from build123d import *

# Parameters (mm, degrees)
BOSS_EXTRUDE1_DEPTH      = 33.02
BOSS_EXTRUDE1_DEPTH_BACK = 33.02
BOSS_EXTRUDE3_DEPTH      = 19.05
BOSS_EXTRUDE3_DEPTH_BACK = 19.05
SKETCH2_6_W              = 38.1
SKETCH2_6_H              = 81.28
SKETCH8_OUTSIDE_W        = 151.232
SKETCH8_OUTSIDE_H        = 112.624
SKETCH8_OUTSIDE_R        = 19.05
CUT_EXTRUDE1_DEPTH       = 81.28
CHAMFER2_SIZE            = 2.54
FILLET2_R                = 33.02
HOLE1_D                  = 25.4


with BuildPart() as part:
    # Sketch2 → Boss-Extrude1 (new, two sides: drawn at the far end of the back side and taken through both)
    with BuildSketch(Plane.XY.offset(-BOSS_EXTRUDE1_DEPTH_BACK)):
        with BuildLine():
            ThreePointArc((-52.324, 0), (-45.330881508, 16.882881508), (-28.448, 23.876))
            Line((-28.448, 23.876), (28.448, 23.876))
            ThreePointArc((28.448, 23.876), (45.330881508, 16.882881508), (52.324, 0))
            Line((52.324, 0), (52.324, -80.264))
            Line((52.324, -80.264), (28.575, -80.264))
            Line((28.575, -80.264), (28.575, -7.874))
            Line((28.575, -7.874), (-28.575, -7.874))
            Line((-28.575, -7.874), (-28.575, -80.264))
            Line((-28.575, -80.264), (-52.324, -80.264))
            Line((-52.324, -80.264), (-52.324, 0))
        make_face()
    extrude(amount=BOSS_EXTRUDE1_DEPTH + BOSS_EXTRUDE1_DEPTH_BACK)

    # Sketch2<6> → Boss-Extrude3 (add, two sides: drawn at the far end of the back side and taken through both)
    with BuildSketch(Plane.XY.offset(-BOSS_EXTRUDE3_DEPTH_BACK)):
        with Locations((0, 64.516)):
            Rectangle(SKETCH2_6_W, SKETCH2_6_H)
    extrude(amount=BOSS_EXTRUDE3_DEPTH + BOSS_EXTRUDE3_DEPTH_BACK)

    # Sketch8 outside → Cut-Extrude1 (cut)
    with BuildSketch(Plane(origin=(0, 105.156, 0), x_dir=(1, 0, 0), z_dir=(0, 1, 0))):
        Rectangle(SKETCH8_OUTSIDE_W, SKETCH8_OUTSIDE_H)
        with Locations(Location((0, 0, 0), (0, 0, 270))):
            Circle(SKETCH8_OUTSIDE_R, mode=Mode.SUBTRACT)
    extrude(amount=-CUT_EXTRUDE1_DEPTH, mode=Mode.SUBTRACT)

    # Chamfer2
    chamfer2_edges = [part.edges().sort_by_distance(p)[0] for p in [
        (0, 105.156, -19.05),
    ]]
    chamfer(chamfer2_edges, length=CHAMFER2_SIZE)

    # Fillet2
    fillet2_edges = [part.edges().sort_by_distance(p)[0] for p in [
        (-40.4495, -80.264, -33.02),
        (40.4495, -80.264, -33.02),
        (40.4495, -80.264, 33.02),
        (-40.4495, -80.264, 33.02),
    ]]
    fillet(fillet2_edges, radius=FILLET2_R - 0.0001)  # a hair under: the kernel refuses the full size

    # Hole1 (through all)
    with Locations(Plane(origin=(52.324, 0, 0), x_dir=(0, 0, -1), z_dir=(1, 0, 0))):
        with Locations((0, -47.244)):
            Hole(HOLE1_D / 2)


solid = part.part
Model file for the job. Use its own axes, mm. A direction names the side the tool comes from. Give positions to 0.01 mm unless a question says otherwise; leave off trailing zeros. Order: outer loops, then holes, each group sorted by start corner. A loop starts at its lowest first (then second) coordinate and runs counter-clockwise, first axis right, second up. Notation, with made-up numbers: (-40, 3.25) - (1, 3.25) arc R23 cw to (1, 19.25) - close; hole circle Ø7 at (74.25, -32). An arc over 180 degrees is marked (long way). Return JSON: item names as keys, results as strings.
1) Cut at C-C, the plane x = 0. Give the cut face in (y, z).
Geometry says:
{"outline": "(-7.87, -33.02) - (23.88, -33.02) - (23.88, -19.05) - (102.62, -19.05) - (105.16, -16.51) - (105.16, 16.51) - (102.62, 19.05) - (23.88, 19.05) - (23.88, 33.02) - (-7.87, 33.02) - close"}
2) Cut at D-D, the plane z = 8. Count the separate pieces of the cut face and the enclosed holes in it, plus the area to 3 significant figures.
Geometry says:
{"separate pieces": "3", "enclosed holes": "0", "area": "8,340 mm²"}
3) 3-axis set-ups, long thin cutter, end or side, ignore diameter. For faces 4 (the cylindrical face through (-11.59, 63.8, -15.12)), 5 (the cylindrical face through (-45.515, 16.696, -0.462)), 6 (the flat face through (-28.575, -36, -8)): which of +Z, -Z, +X, -X, +Y, -Y reach the whole face in a straight line?
Geometry says:
{"face 4": "+Y", "face 5": "+Z, -Z, -X, +Y", "face 6": "+Z, -Z, -Y"}
4) Probe line 1 (X direction, y = -24, z = -19) (3 decimals); line 2 (X direction, y = 80, z = -0.5); line 3 (Z direction, x = -39.5, y = -52). List the from-to ranges inside material, lowest first. Write a range as from..to.
Geometry says:
{"line 1": "-52.324..-28.575, 28.575..52.324", "line 2": "-19.04..19.04", "line 3": "-32.68..-11.78, 11.78..32.68"}
5) Pull direction Y, two halves, no side cores. Call faces 1 (the cylindrical face through (-40.62, -58.51, 5.86)), 2 (the flat face through (52.324, -31, 0)), 3 (the cylindrical face through (-40.616, -70.335, -23.604)): pulls with the +Y half, pulls with the -Y half, needs draft (parallel to the pull), parting line crosses it, or undercut.
Geometry says:
{"face 1": "undercut", "face 2": "needs draft", "face 3": "pulls with the -Y half"}
6) Cut at A-A, the plane y = -24. Give the cut face in (x, z) (3 decimals).
Geometry says:
{"outline": "(-52.324, -33.02) - (-28.575, -33.02) - (-28.575, 33.02) - (-52.324, 33.02) - close; (28.575, -33.02) - (52.324, -33.02) - (52.324, 33.02) - (28.575, 33.02) - close"}
7) Flat gauge pins, fed straight in: P1, Ø12, axis at x = 16, z = -9.5, coming from the +Y side; P2, Ø8, axis at y = 67, z = 16, coming from the +X side; P3, Ø4, axis at y = 84.5, z = 9.5, coming from the +X side; P4, Ø4, axis at x = 36.5, z = -3.5, coming from the -Y side. Where does each tip first touch, or does it go through?
Geometry says:
{"P1": "y = 105.16", "P2": "x = 14.8", "P3": "x = 17.51", "P4": "y = -80.23"}
